Check sheet for the drawn part. Datum: minimum x, y, z corner. Units: mm. Give positions to 0.01 mm unless a question says otherwise; leave off trailing zeros. Order: outer loops, then holes, each group sorted by start corner. A loop starts at its lowest first (then second) coordinate and runs counter-clockwise, first axis right, second up.
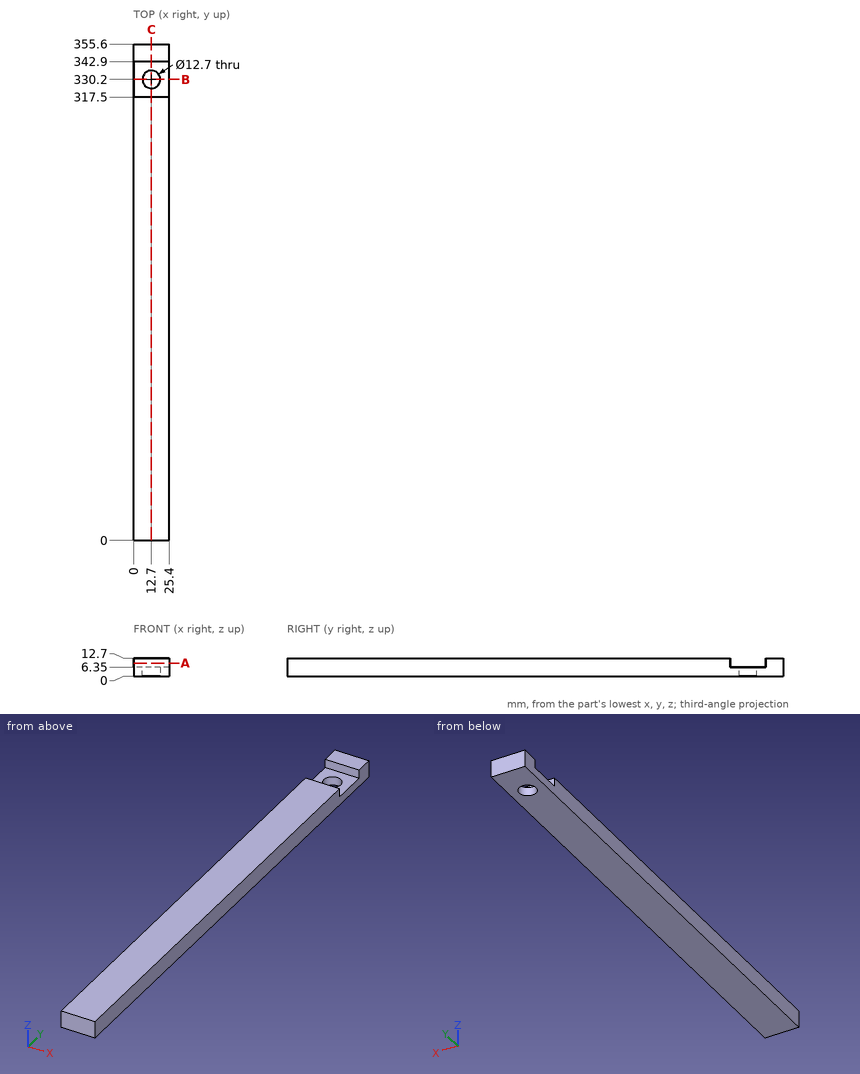
(1) Scan lines: line 1 (X direction, y = 330.2, z = 3.75); line 2 (Y direction, x = 12.7, z = 4.75); line 3 (Y direction, x = 23.75, z = 10.75). Record each from-to range of solid material in increasing order.
Solved:
line 1: x = 0 to 6.35, 19.05 to 25.4
line 2: y = 0 to 323.85, 336.55 to 355.6
line 3: y = 0 to 317.5, 342.9 to 355.6
(2) Section check A-A, the plane z = 9.25. Enter the section's corners in (x, y), then the cut area to 3 significant figures.
Solved:
outline: (0, 0) - (25.4, 0) - (25.4, 317.5) - (0, 317.5) - close; (0, 342.9) - (25.4, 342.9) - (25.4, 355.6) - (0, 355.6) - close
area: 8,390 mm2
(3) Section check C-C, the plane x = 12.7. Enter the section's corners in (y, z), then the cut area to 3 significant figures.
Solved:
outline: (0, 0) - (323.85, 0) - (323.85, 6.35) - (317.5, 6.35) - (317.5, 12.7) - (0, 12.7) - close; (336.55, 0) - (355.6, 0) - (355.6, 12.7) - (342.9, 12.7) - (342.9, 6.35) - (336.55, 6.35) - close
area: 4,270 mm2
(4) Go/stop test with a flat-tipped pin: pin 1 (14.5 mm diameter, centred on x = 12.7, y = 330.2, fed in from +Z). Record where the tip stops, or that it passes through.
Solved:
pin 1: stops at z = 6.35
(5) Section check B-B, the plane y = 330.2. Enter the section's corners in (x, z).
Solved:
outline: (0, 0) - (6.35, 0) - (6.35, 6.35) - (0, 6.35) - close; (19.05, 0) - (25.4, 0) - (25.4, 6.35) - (19.05, 6.35) - close
